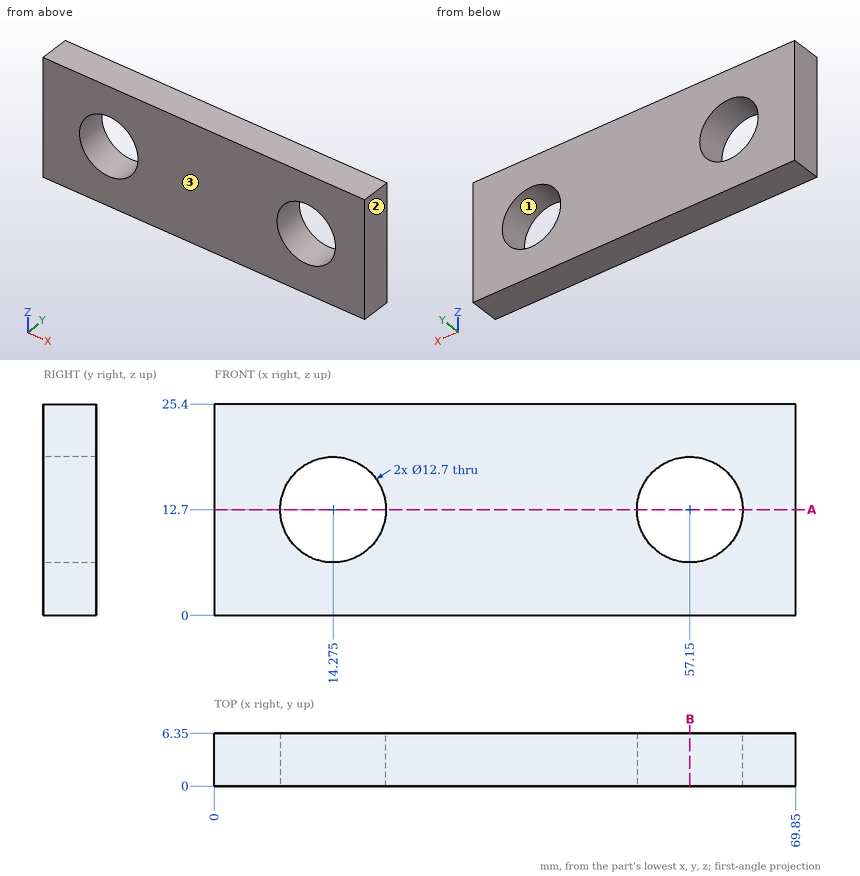
Design review of the part shown in the three views and the two pictorial views. Dimensions are in mm from the part's minimum x, y and z. Round coordinates to 2 decimals unless told otherwise and drop trailing zeros. Loops run counter-clockwise (first coordinate to the right, second up) from the corner with the lowest first, then second, coordinate; pieces in that order, holes last.
(1) We need section A-A (z = 12.7). State how many separate pieces and enclosed holes the cut face has, plus the area to 3 significant figures.
Returned:
separate pieces: 3
enclosed holes: 0
area: 282 mm2
(2) Clearance check with flat-ended pins moving along their axes: P1, Ø2, axis at y = 1, z = 14.5, coming from the -X side; P2, Ø11.5, axis at x = 57.15, z = 12.7, coming from the -Y side. State where each tip first meets the part, or that it passes through.
Returned:
P1: stops at x = 0
P2: passes through
(3) Wall thickness on line 1 along Z through (x, y) = (13.5, 2.5); line 2 along Z through (x, y) = (20, 3.75) (1 decimal); line 3 along X through (y, z) = (5.5, 15): over which ranges is each line inside the solid? List them lowest first.
Returned:
line 1: z = 0 to 6.4, 19 to 25.4
line 2: z = 0 to 10, 15.4 to 25.4
line 3: x = 0 to 8.36, 20.19 to 51.23, 63.07 to 69.85
(4) We need section B-B (x = 57.15). Give the boundary of the cut face in (y, z).
Returned:
outline: (0, 0) - (6.35, 0) - (6.35, 6.35) - (0, 6.35) - close; (0, 19.05) - (6.35, 19.05) - (6.35, 25.4) - (0, 25.4) - close
(5) Mouldability with a two-part tool opening along X and no side actions: class the marked faces 1, 2 and 3 as released by +X, released by -X, zero draft, split by the parting line, or undercut.
Returned:
face 1: undercut
face 2: released by +X
face 3: zero draft
